```python
from build123d import *

# Parameters (mm, degrees)
BOSS_EXTRUDE1_DEPTH = 4.75
SKETCH1_4_R         = 4.75
BOSS_EXTRUDE2_DEPTH = 50
SKETCH3_R           = 14.5
BOSS_EXTRUDE3_DEPTH = 3
CUT_EXTRUDE1_REACH  = 56.75
SKETCH4_R           = 2.5
SKETCH5_R           = 2.5
CUT_EXTRUDE2_DEPTH  = 5
SKETCH6_R           = 2.5
BOSS_EXTRUDE5_DEPTH = 5
BOSS_EXTRUDE6_REACH = 56.75
SKETCH7_R           = 4.825
SKETCH8_R           = 2
CUT_EXTRUDE3_DEPTH  = 3


with BuildPart() as part:
    # Sketch1 → Boss-Extrude1 (new body)
    with BuildSketch(Plane(origin=(0, 0, 0), x_dir=(1, 0, 0), z_dir=(0, 1, 0))):
        with BuildLine():
            Line((0, 14.5), (-122.9, 7.5))
            ThreePointArc((-122.9, 7.5), (-130.4, 0), (-122.9, -7.5))
            Line((-122.9, -7.5), (0, -14.5))
            Line((0, -14.5), (122.9, -7.5))
            ThreePointArc((122.9, -7.5), (130.4, 0), (122.9, 7.5))
            Line((122.9, 7.5), (0, 14.5))
        make_face()
    extrude(amount=BOSS_EXTRUDE1_DEPTH)

    # Sketch1<4> → Boss-Extrude2 (add)
    with BuildSketch(Plane(origin=(0, 0, 0), x_dir=(1, 0, 0), z_dir=(0, 1, 0))):
        Circle(SKETCH1_4_R)
    extrude(amount=-BOSS_EXTRUDE2_DEPTH)

    # Sketch3 → Boss-Extrude3 (add)
    with BuildSketch(Plane.XZ):
        Circle(SKETCH3_R)
    extrude(amount=BOSS_EXTRUDE3_DEPTH)

    # Sketch4 → Cut-Extrude1 (cut, up to next)
    with BuildSketch(Plane(origin=(0, 4.75, 0), x_dir=(1, 0, 0), z_dir=(0, 1, 0)), mode=Mode.PRIVATE) as cut_extrude1_sk1:
        with Locations((111.778793877, 0)):
            Circle(SKETCH4_R)
    cut_extrude1_tool1 = extrude(cut_extrude1_sk1.sketch, amount=-CUT_EXTRUDE1_REACH, mode=Mode.PRIVATE) & part.part
    add(cut_extrude1_tool1.solids().sort_by_distance((111.778794, 4.75, 0))[0], mode=Mode.SUBTRACT)
    # Sketch4 → Cut-Extrude1 (cut, up to next)
    with BuildSketch(Plane(origin=(0, 4.75, 0), x_dir=(1, 0, 0), z_dir=(0, 1, 0)), mode=Mode.PRIVATE) as cut_extrude1_sk2:
        with Locations((-118.05968216, 0)):
            Circle(SKETCH4_R)
    cut_extrude1_tool2 = extrude(cut_extrude1_sk2.sketch, amount=-CUT_EXTRUDE1_REACH, mode=Mode.PRIVATE) & part.part
    add(cut_extrude1_tool2.solids().sort_by_distance((-118.059682, 4.75, 0))[0], mode=Mode.SUBTRACT)

    # Sketch5 → Cut-Extrude2 (cut)
    with BuildSketch(Plane(origin=(0, 4.75, 0), x_dir=(1, 0, 0), z_dir=(0, 1, 0))):
        with Locations((-118.05968216, 0)):
            Circle(SKETCH5_R)
        with Locations((118.05968216, 0)):
            Circle(SKETCH5_R)
    extrude(amount=-CUT_EXTRUDE2_DEPTH, mode=Mode.SUBTRACT)

    # Sketch6 → Boss-Extrude5 (add)
    with BuildSketch(Plane(origin=(0, 4.75, 0), x_dir=(1, 0, 0), z_dir=(0, 1, 0))):
        with Locations((111.778793877, 0)):
            Circle(SKETCH6_R)
    extrude(amount=-BOSS_EXTRUDE5_DEPTH)

    # Sketch7 → Boss-Extrude6 (add, up to next)
    with BuildSketch(Plane(origin=(0, -50, 0), x_dir=(-1, 0, 0), z_dir=(0, -1, 0)), mode=Mode.PRIVATE) as boss_extrude6_sk1:
        Circle(SKETCH7_R)
    boss_extrude6_tool1 = extrude(boss_extrude6_sk1.sketch, amount=-BOSS_EXTRUDE6_REACH, mode=Mode.PRIVATE) - part.part
    add(boss_extrude6_tool1.solids().sort_by_distance((0, -50, 0))[0])

    # Sketch8 → Cut-Extrude3 (cut)
    with BuildSketch(Plane.XZ.offset(50)):
        Circle(SKETCH8_R)
    extrude(amount=-CUT_EXTRUDE3_DEPTH, mode=Mode.SUBTRACT)


solid = part.part
```
Check sheet for the modelled part. Datum: model origin and axes. Units: mm. A direction names the side the tool comes from. Round coordinates to 2 decimals unless told otherwise and drop trailing zeros. Order: outer loops, then holes, each group sorted by start corner. A loop starts at its lowest first (then second) coordinate and runs counter-clockwise, first axis right, second up. Notation, with made-up numbers: (-39.5, 86) -> (13.5, 86) arc R11 ccw to (13.5, 99) -> close; hole circle Ø1 at (-20, 39). An arc over 180 degrees is marked (long way). One line per item, written item: value. Start each with the question number.
Q1. Cross-section at C-C (x = 97.5). Record the boundary of the cut face in (y, z).
Q2. Gauge pin test, flat ends, axial feed: pin 1 Ø12 at (x, z) = (78.5, 1.5) entering from -Y; pin 2 Ø12 at (x, z) = (-12.5, 8) entering from -Y; pin 3 Ø4 at (x, z) = (112.5, -0.5) entering from -Y; pin 4 Ø3 at (x, z) = (0, -1) entering from -Y. Record the tip position at first contact, or that the pin passes through.
Q3. Cross-section at B-B (x = 35). Record the boundary of the cut face in (y, z), and give its area (3 significant figures).
Q4. Thickness scan on line 1 (X direction, y = 2.3, z = 0); line 2 (Y direction, x = 16, z = -10.25); line 3 (Z direction, x = 0, y = -48.55) (3 decimals). Record the ranges inside material, lowest first.
Q5. Mould release check, pull along X, two halves, no side actions. Record for faces 1 (the face through (120.444, 2.408, -0.751)), 2 (the face through (-62.31, 2.34, 10.95)), 3 (the face through (-4.6, -26.83, -1.45)): pulls with the +X half, pulls with the -X half, needs draft (parallel to the pull), parting line crosses it, or undercut.
Q6. Cross-section at A-A (y = -14.5). Record the boundary of the cut face in (x, z) (3 decimals), and give its area (3 significant figures).
Q7. Set-up check for faces 4 (the face through (-60.59, 2.34, -11.05)), 5 (the face through (6, -3, 0)), 6 (the face through (112, -0.25, 0)): record each of +Z, -Z, +X, -X, +Y, -Y from which the full face is reachable in a straight line by a thin tool's end or side.
Completed:
1. outline: (0, -8.95) -> (4.75, -8.95) -> (4.75, 8.95) -> (0, 8.95) -> close
2. pin 1: stops at y = 0
2. pin 2: stops at y = -3
2. pin 3: stops at y = -0.25
2. pin 4: stops at y = -50
3. outline: (0, -12.51) -> (4.75, -12.51) -> (4.75, 12.51) -> (0, 12.51) -> close
3. area: 119 mm²
4. line 1: x = -130.4 to -120.56, -115.56 to 115.56, 120.56 to 130.4
4. line 2: y = 0 to 4.75
4. line 3: z = -4.825 to -2, 2 to 4.825
5. face 1: undercut
5. face 2: pulls with the -X half
5. face 3: parting line crosses it
6. outline: circle Ø9.65 at (0, 0)
6. area: 73.1 mm²
7. face 4: -Z, -X, +Y, -Y
7. face 5: -Y
7. face 6: +Z, -Z, +X, -Y
